Geometry check sheet. Reference: the model listing, model coordinates, mm. Face numbers are marked on the shaded views. A direction names the side the tool comes from. Round coordinates to 2 decimals unless told otherwise and drop trailing zeros. Order: outer loops, then holes, each group sorted by start corner. A loop starts at its lowest first (then second) coordinate and runs counter-clockwise, first axis right, second up. Notation, with made-up numbers: (48.25, 31) - (100.25, 31) arc R4 cw to (100.25, 36) - close; hole circle Ø1 at (-12.5, -35.75). An arc over 180 degrees is marked (long way). One line per question, with ' | ' between items. Start each with the question number.
Q1. Gauge pin test, flat ends, axial feed: P1, Ø1, axis at x = -16.5, y = 2.5, coming from the -Z side; P2, Ø3.5, axis at x = -23, y = 0.5, coming from the -Z side; P3, Ø1.5, axis at x = -22.5, y = 0.5, coming from the +Z side; P4, Ø2, axis at y = 1.5, z = -0.5, coming from the -X side. Record the tip position at first contact, or that the pin passes through.
Q2. Mould release check, pull along X, two halves, no side actions. Record for the marked faces 1 and 2: +X half, -X half, draft (parallel to the pull), parting line (faces both ways), or undercut.
Q3. Material ranges on line 1 along Y through (x, z) = (-17.25, -2); line 2 along X through (y, z) = (2.2, -7.5); line 3 along Z through (x, y) = (-17.75, 1.05), recorded low to high.
Q4. Sectioned sample at A-A, the plane z = -10. Enter the section's corners in (x, y), then the cut area to 3 significant figures.
Q5. Sectioned sample at D-D, the plane x = -16.5. Enter the section's corners in (y, z), then the cut area to 3 significant figures.
Q6. Sectioned sample at B-B, the plane z = 0. Enter the section's corners in (x, y).
Q7. Sectioned sample at C-C, the plane y = 0.4. Enter the section's corners in (x, z), then the cut area to 3 significant figures.
Q8. Tool access check on the marked faces 3 and 4. Record the directions out of +Z, -Z, +X, -X, +Y, -Y that give a thin tool (end or side, any length) a straight path to the whole face; none if there is none.
Autodesk Inventor part; units mm, degrees
ref_plane "YZ Plane" through (0, 0, 0) normal (1, 0, 0) x (0, 1, 0)
ref_plane "XZ Plane" through (0, 0, 0) normal (0, 1, 0) x (-1, 0, 0)
ref_plane "XY Plane" through (0, 0, 0) normal (0, 0, 1) x (1, 0, 0)
sketch "Sketch1" plane through (0, 0, 0) normal (0, 1, 0) x (-1, 0, 0)
  circle A0 centre (0, 0) radius 14.5
  circle A1 centre (0, 0) radius 16
  line L0 (0, 16) -> (0, -16)
  line L1 (14.5, 5.0206) -> (21.5, 5.0206)
  line L2 (21.5, 5.0206) -> (21.5, -4.9794)
  line L3 (21.5, -4.9794) -> (14.5, -4.9794)
  line L4 (14.5, -4.9794) -> (14.5, 5.0206)
  point P0 (14.5, 0.0206)
  point P1 (15.2054, -4.9794)
  point P2 (15.1919, 5.0206)
  point P3 (0, 14.5)
  point P4 (0, -14.5)
  dimension "d0" = 29
  dimension "d1" = 32
  dimension "d2" = 5
  dimension "d13" = 7
extrude "Extrusion1" add sketch "Sketch1" along normal blind 1.5 contours L4 L3 A1 L0 A0 | L4 L1 A1 L3 | A0 L0 A1 L1 L4 | A1 L1 L2 L3
sketch "Sketch2" plane through (-21.5, 0, -4.9794) normal (-1, 0, 0) x (0, 0, 1)
  line L0 (-5.3921, 3.75) -> (15.5709, 3.75)
  line L1 (15.5709, 3.75) -> (15.5709, -2.25)
  line L2 (15.5709, -2.25) -> (-5.3921, -2.25)
  line L3 (-5.3921, -2.25) -> (-5.3921, 3.75)
  line L4 (0, 0) -> (0, 1.5)
  point P0 (4.9794, 0)
  point P1 (5.0894, 3.75)
  point P2 (0, 0.75)
  dimension "d5" = 6
  dimension "d6" = 3
extrude "Extrusion2" add sketch "Sketch2" along normal blind 1.5
sketch "Sketch3" plane through (-23, 0, -4.9794) normal (-1, 0, 0) x (0, 0, 1)
  line L0 (15.5709, 3.75) -> (-5.3921, 3.75)
  line L1 (15.5709, -2.25) -> (15.5709, 3.75)
  line L2 (-5.3921, 3.75) -> (15.5709, 3.75)
  line L3 (15.5709, 3.75) -> (15.5709, 2.75)
  line L4 (15.5709, 2.75) -> (-5.3921, 2.75)
  line L5 (-5.3921, 2.75) -> (-5.3921, 3.75)
  line L6 (-5.3921, -2.25) -> (15.5709, -2.25)
  line L7 (15.5709, -2.25) -> (15.5709, -1.25)
  line L8 (15.5709, -1.25) -> (-5.3921, -1.25)
  line L9 (-5.3921, -1.25) -> (-5.3921, -2.25)
  point P0 (4.9794, 0)
  point P1 (15.5709, -2.25)
  dimension "d9" = 1
  dimension "d10" = 1
extrude "Extrusion3" add sketch "Sketch3" along normal blind 1.5
properties part number "holder"
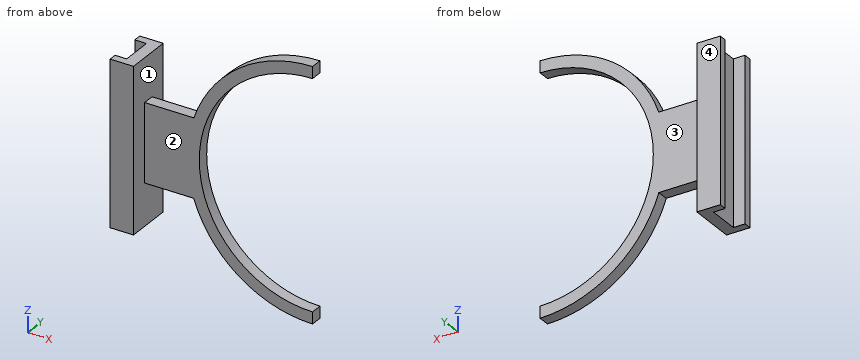
Determined:
1) P1: passes through | P2: stops at z = -10.37 | P3: stops at z = 10.59 | P4: stops at x = -23
2) face 1: undercut | face 2: draft
3) line 1: y = 0 to 1.5 | line 2: x = -23 to -21.5 | line 3: z = -4.98 to 5.02
4) outline: (-24.5, -2.25) - (-21.5, -2.25) - (-21.5, 3.75) - (-24.5, 3.75) - (-24.5, 2.75) - (-23, 2.75) - (-23, -1.25) - (-24.5, -1.25) - close; (-12.49, 0) - (-10.5, 0) - (-10.5, 1.5) - (-12.49, 1.5) - close | area: 15.0 mm2
5) outline: (0, -4.98) - (1.5, -4.98) - (1.5, 5.02) - (0, 5.02) - close | area: 15.0 mm2
6) outline: (-24.5, -2.25) - (-21.5, -2.25) - (-21.5, 0) - (-14.5, 0) - (-14.5, 1.5) - (-21.5, 1.5) - (-21.5, 3.75) - (-24.5, 3.75) - (-24.5, 2.75) - (-23, 2.75) - (-23, -1.25) - (-24.5, -1.25) - close
7) outline: (-23, -10.37) - (-21.5, -10.37) - (-21.5, -4.98) - (-15.21, -4.98) arc R16 ccw to (0, -16) - (0, -14.5) arc R14.5 cw to (0, 14.5) - (0, 16) arc R16 ccw to (-15.19, 5.02) - (-21.5, 5.02) - (-21.5, 10.59) - (-23, 10.59) - close | area: 161 mm2
8) face 3: +Z, -Z, +X, +Y | face 4: +Z, -Z, +X, -X, +Y
